Here's how the part is built. I have some questions about the finished solid (model axes, mm). Face numbers are marked on the shaded views. Coordinates: 2 decimals unless noted, no trailing zeros. Order: outer loops, then holes, each group sorted by start corner. A loop starts at its lowest first (then second) coordinate and runs counter-clockwise, first axis right, second up.
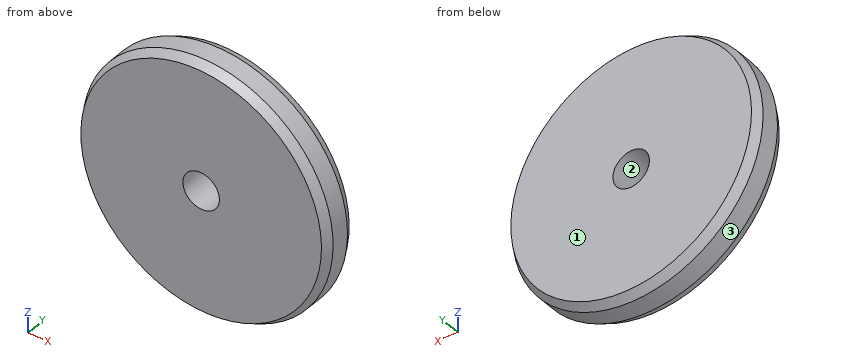
```python
from build123d import *

# Parameters (mm, degrees)
SKETCH_1_R               = 17.5
EXTRUDE_1_DEPTH          = 5
CUT_EXTRUDE_1_DEPTH      = 26.248762346
CUT_EXTRUDE_1_DEPTH_BACK = 26.248762346
SKETCH_2_R               = 2.55
CHAMFER_1_SIZE           = 1.2
CHAMFER_1_SIZE2          = 0.692820323


with BuildPart() as part:
    # 스케치1 → 보스-돌출1 (new body)
    with BuildSketch(Plane(origin=(0, 0, 0), x_dir=(1, 0, 0), z_dir=(0, 1, 0))):
        with Locations(Location((0, 0, 0), (0, 0, 270))):
            Circle(SKETCH_1_R)
    extrude(amount=EXTRUDE_1_DEPTH)

    # 스케치2 → 컷-돌출1 (cut, two sides: drawn at the far end of the back side and taken through both)
    with BuildSketch(Plane(origin=(0, 5, 0), x_dir=(1, 0, 0), z_dir=(0, 1, 0)).offset(-CUT_EXTRUDE_1_DEPTH_BACK)):
        with Locations(Location((0, 0, 0), (0, 0, 270))):
            Circle(SKETCH_2_R)
    extrude(amount=CUT_EXTRUDE_1_DEPTH + CUT_EXTRUDE_1_DEPTH_BACK, mode=Mode.SUBTRACT)

    # 모따기1
    chamfer_1_edges = [part.edges().sort_by_distance(p)[0] for p in [
        (0, 0, -17.5),
        (0, 5, -17.5),
    ]]
    chamfer_1_side = [part.faces().sort_by_distance(p)[0] for p in [
        (0, 2.5, -17.5),
    ]]
    chamfer(chamfer_1_edges, length=CHAMFER_1_SIZE, length2=CHAMFER_1_SIZE2, reference=chamfer_1_side[0])


solid = part.part
```
Q1. If we section it at A-A on z = 0: Write out the boundary of the cut face in (x, y), then the cut area to 3 significant figures.
Q2. If we section it at C-C on y = 2.15: Write out the boundary of the cut face in (x, z), then the cut area to 3 significant figures.
Q3. We'd pull the mould along X, two halves only. Please class the marked faces 1, 2 and 3: pulls with the +X half, pulls with the -X half, needs draft (parallel to the pull), parting line crosses it, or undercut.
Q4. I need wall thicknesses on L1, parallel to X at y = 2.2, z = 0; L2, parallel to X at y = 2.2, z = 2; L3, parallel to Z at x = -2, y = 4.05. Which ranges of each line are inside material? Lowest first, please.
Q5. Will these pins go through, and if not, where does the flat tip stop? pin 1 (1 mm diameter, centred on y = 4, z = 5.5, fed in from -X); pin 2 (1.5 mm diameter, centred on y = 1.5, z = 5, fed in from -X).
Q6. If we section it at B-B on x = 0: Write out the boundary of the cut face in (y, z).
Reply:
1. outline: (-17.5, 1.2) - (-16.81, 0) - (-2.55, 0) - (-2.55, 5) - (-16.81, 5) - (-17.5, 3.8) - close; (2.55, 0) - (16.81, 0) - (17.5, 1.2) - (17.5, 3.8) - (16.81, 5) - (2.55, 5) - close
1. area: 148 mm2
2. outline: circle Ø35 at (0, 0); hole circle Ø5.1 at (0, 0)
2. area: 942 mm2
3. face 1: needs draft
3. face 2: undercut
3. face 3: parting line crosses it
4. L1: x = -17.5 to -2.55, 2.55 to 17.5
4. L2: x = -17.39 to -1.58, 1.58 to 17.39
4. L3: z = -17.24 to -1.58, 1.58 to 17.24
5. pin 1: stops at x = -16.76
5. pin 2: stops at x = -16.98
6. outline: (0, -16.81) - (1.2, -17.5) - (3.8, -17.5) - (5, -16.81) - (5, -2.55) - (0, -2.55) - close; (0, 2.55) - (5, 2.55) - (5, 16.81) - (3.8, 17.5) - (1.2, 17.5) - (0, 16.81) - close
